Design review of the part built by this model. Coordinates are the model's own, in mm. A direction names the side the tool comes from. Coordinates: 2 decimals unless noted, no trailing zeros. Write each loop counter-clockwise with the first axis right and the second up, starting at its lowest first coordinate (ties: lowest second). Pieces come first, ordered by that corner, then holes. Notation, with made-up numbers: (58.5, -14.75) - (107.5, -14.75) arc R30 ccw to (107.5, 9.25) - close; hole circle Ø4 at (43, 66). An arc over 180 degrees is marked (long way). Use a Markdown table: item, result.
from build123d import *
from OCP.BRepFilletAPI import BRepFilletAPI_MakeFillet

# Parameters (mm, degrees)
BOSS_EXTRUDE1_DEPTH = 11.5
SKETCH1_3_W         = 5.5
SKETCH1_3_H         = 3.2
BOSS_EXTRUDE2_DEPTH = 8.4
CUT_EXTRUDE1_DEPTH  = 1.8
SKETCH5_3_W         = 2.721866022
SKETCH5_3_H         = 2.25
CUT_EXTRUDE2_DEPTH  = 29.993318196
FILLET1_R           = 4.2
FILLET1_R_2         = 1.125
FILLET1_R_3         = 1
FILLET1_R_4         = 0.5
CUT_EXTRUDE12_DEPTH = 1.8


with BuildPart() as part:
    # Sketch1 → Boss-Extrude1 (new body)
    with BuildSketch(Plane.XY):
        Polygon((5.5, 7.95), (5.5, 0), (5.5, -3.2), (6.8, -3.2), (6.8, 6.65), (12.7, 6.65), (12.7, 7.95), align=None)
        Polygon((19.9, 7.95), (12.7, 7.95), (12.7, 6.65), (18.6, 6.65), (18.6, -3.2), (19.9, -3.2), (19.9, 0), align=None)
    extrude(amount=BOSS_EXTRUDE1_DEPTH)

    # Sketch1<3> → Boss-Extrude2 (add)
    with BuildSketch(Plane.XY):
        with Locations((2.75, -1.6)):
            Rectangle(SKETCH1_3_W, SKETCH1_3_H)
        with Locations((22.65, -1.6)):
            Rectangle(SKETCH1_3_W, SKETCH1_3_H)
    extrude(amount=BOSS_EXTRUDE2_DEPTH)

    # Sketch5 → Cut-Extrude1 (cut)
    with BuildSketch(Plane(origin=(0, 0, 0), x_dir=(1, 0, 0), z_dir=(0, 1, 0))):
        Polygon((3.478202851, -1.61261316), (1.3, -2.596789569), (1.3, -5.354715804), (3.478202851, -6.338892213), (5.5, -5.201401594), (5.5, -5.100752687), (2.778133978, -5.100752687), (2.778133978, -2.850752687), (5.5, -2.850752687), (5.5, -2.750103779), align=None)
        Polygon((19.9, -5.100752687), (19.9, -5.201401594), (21.921797149, -6.338892213), (24.1, -5.354715804), (24.1, -2.596789569), (21.921797149, -1.61261316), (19.9, -2.750103779), (19.9, -2.850752687), (22.621866022, -2.850752687), (22.621866022, -5.100752687), align=None)
    extrude(amount=-CUT_EXTRUDE1_DEPTH, mode=Mode.SUBTRACT)

    # Sketch5<3> → Cut-Extrude2 (cut, through all)
    with BuildSketch(Plane(origin=(0, 0, 0), x_dir=(1, 0, 0), z_dir=(0, 1, 0))):
        Polygon((2.778133978, -2.850752687), (2.778133978, -3.975752687), (2.778133978, -5.100752687), (5.5, -5.100752687), (5.5, -2.850752687), align=None)
        with Locations((21.260933011, -3.975752687)):
            Rectangle(SKETCH5_3_W, SKETCH5_3_H)
    extrude(amount=-CUT_EXTRUDE2_DEPTH, mode=Mode.SUBTRACT)

    # Fillet1
    fillet1_edges_1 = [part.edges().sort_by_distance(p)[0] for p in [
        (0, -1.6, 0),
        (0, -1.6, 8.4),
        (25.4, -1.6, 8.4),
        (25.4, -1.6, 0),
    ]]
    fillet1_edges_2 = [part.edges().sort_by_distance(p)[0] for p in [
        (2.778133978, -2.5, 5.100752687),
        (2.778133978, -2.5, 2.850752687),
        (22.621866022, -2.5, 2.850752687),
        (22.621866022, -2.5, 5.100752687),
    ]]
    fillet1_edges_3 = [part.edges().sort_by_distance(p)[0] for p in [
        (5.5, 7.95, 5.75),
        (19.9, 7.95, 5.75),
        (18.6, 6.65, 5.75),
        (6.8, 6.65, 5.75),
    ]]
    fillet1_edges_4 = [part.edges().sort_by_distance(p)[0] for p in [
        (5.5, 0, 6.800700797),
        (19.9, 0, 6.800700797),
        (19.9, 0, 1.37505189),
        (5.5, 0, 1.37505189),
    ]]
    fillet1 = BRepFilletAPI_MakeFillet(part.part.solid().wrapped)
    for e in fillet1_edges_1:
        fillet1.Add(FILLET1_R - 0.0001, e.wrapped)
    for e in fillet1_edges_2:
        fillet1.Add(FILLET1_R_2 - 0.0001, e.wrapped)
    for e in fillet1_edges_3:
        fillet1.Add(FILLET1_R_3 - 0.0001, e.wrapped)
    for e in fillet1_edges_4:
        fillet1.Add(FILLET1_R_4 - 0.0001, e.wrapped)
    add(Compound.cast(fillet1.Shape()), mode=Mode.REPLACE)  # a hair under: the kernel refuses the full size

    # Sketch6 → Cut-Extrude12 (cut)
    with BuildSketch(Plane.XZ.offset(3.2)):
        Polygon((19.9, 5.100752687), (19.9, 2.850752687), (19.9, 2.350752687), (18.327658743, 2.350752687), (18.327658743, 5.600752687), (19.9, 5.600752687), align=None)
        Polygon((5.5, 5.600752687), (5.5, 5.100752687), (5.5, 2.850752687), (5.5, 2.350752687), (6.8, 2.350752687), (6.8, 5.600752687), align=None)
    extrude(amount=-CUT_EXTRUDE12_DEPTH, mode=Mode.SUBTRACT)


solid = part.part
(1) Take a section at C-C on z = 3.25. Write out the cut boundary in (x, y).
Determined:
| item | result |
|---|---|
| outline | (0.11, -3.2) - (3.04, -3.2) - (3.04, -1.8) - (1.3, -1.8) - (1.3, 0) - (0.11, 0) - close; (5.5, -1.4) - (6.8, -1.4) - (6.8, 5.65) arc R1 cw to (7.8, 6.65) - (17.6, 6.65) arc R1 cw to (18.6, 5.65) - (18.6, -1.4) - (19.9, -1.4) - (19.9, 6.95) arc R1 ccw to (18.9, 7.95) - (6.5, 7.95) arc R1 ccw to (5.5, 6.95) - close; (22.36, -3.2) - (25.29, -3.2) - (25.29, 0) - (24.1, 0) - (24.1, -1.8) - (22.36, -1.8) - close |
(2) For pin 1 (1.5 mm diameter, centred on y = 6.5, z = 1.5, fed in from +X); pin 2 (0.6 mm diameter, centred on x = 19, z = 4, fed in from -Y); pin 3 (5 mm diameter, centred on x = 11, z = 6, fed in from -Y); pin 4 (1.5 mm diameter, centred on x = 8.5, y = -1.5, fed in from -Z), all flat-tipped, find the tip position at first contact; note any pin that passes through.
Determined:
| item | result |
|---|---|
| pin 1 | x = 19.9 |
| pin 2 | y = -1.4 |
| pin 3 | y = 6.65 |
| pin 4 | through |
(3) Take a section at A-A on y = 2.5. Write out the cut boundary in (x, z), and give its area (3 significant figures).
Determined:
| item | result |
|---|---|
| outline | (5.5, 0) - (6.8, 0) - (6.8, 11.5) - (5.5, 11.5) - close; (18.6, 0) - (19.9, 0) - (19.9, 11.5) - (18.6, 11.5) - close |
| area | 29.9 mm2 |
(4) For L1, parallel to X at y = 3, z = 6; L2, parallel to Y at x = 3, z = 6; L3, parallel to Y at x = 21.25, z = 6.25, list the stretches that pass through material, from the lowest coordinate up. Write a range as from..to.
Determined:
| item | result |
|---|---|
| L1 | 5.5..6.8, 18.6..19.9 |
| L2 | -3.2..-1.8 |
| L3 | -3.2..0 |
(5) Draft analysis for pull direction Z (two halves, no side actions). For faces 1 (the cylindrical face through (24.14, -1.58, 1.2)), 2 (the flat face through (2, 0, 6)), 3 (the flat face through (20.897, -0.889, 5.762)), state which applies: +Z half, -Z half, draft (parallel to the pull), parting line (faces both ways), or undercut.
Determined:
| item | result |
|---|---|
| face 1 | -Z half |
| face 2 | draft |
| face 3 | undercut |
(6) Machinability: for faces 4 (the cylindrical face through (18.299, 6.365, 5.83)), 5 (the flat face through (24.1, -1, 4)), 6 (the cylindrical face through (22.284, -2.51, 4.78)), which of the approach directions +Z, -Z, +X, -X, +Y, -Y give a long, thin tool a straight path to every point of the face, cutting with its end or side? Answer none if there is none.
Determined:
| item | result |
|---|---|
| face 4 | +Z, -Z, -Y |
| face 5 | +Y |
| face 6 | +Y, -Y |
(7) Take a section at B-B on y = -0.5. State how many separate pieces and enclosed holes the cut face has, and give its area (3 significant figures).
Determined:
| item | result |
|---|---|
| separate pieces | 2 |
| enclosed holes | 2 |
| area | 76.3 mm2 |
(8) Take a section at D-D on x = 5.25. Write out the cut boundary in (y, z), and give its area (3 significant figures).
Determined:
| item | result |
|---|---|
| outline | (-3.2, 0) - (0.07, 0) - (0.07, 2.61) - (-1.8, 2.61) - (-1.8, 2.85) - (-3.2, 2.85) - close; (-3.2, 5.1) - (-1.8, 5.1) - (-1.8, 5.34) - (0.07, 5.34) - (0.07, 8.4) - (-3.2, 8.4) - close |
| area | 19.2 mm2 |
